Study the drawing (mm; zero at the part's minimum x, y, z) and answer. A direction names the side the tool comes from. Coordinates: 2 decimals unless noted, no trailing zeros. Loops run counter-clockwise (first coordinate to the right, second up) from the corner with the lowest first, then second, coordinate; pieces in that order, holes last. Notation, with made-up numbers: (55, -35.5) -> (64, -35.5) arc R13 ccw to (64, -25.5) -> close; hole circle Ø10 at (58, 55.5). An arc over 180 degrees is marked (long way). Answer as a JSON object with one key per item and string values. Group by question number.
Q1. The part is cut by section A-A on y = 7. Write down the section's boundary in (x, z).
Q2. The part is cut by section D-D on z = 46. Write down the section's boundary in (x, y) (3 decimals), and give its area (3 significant figures).
Q3. Straight lines are drawn through the part: line 1 along Z through (x, y) = (9.25, 2); line 2 along Z through (x, y) = (6.5, 3.75); line 3 along X through (y, z) = (5.5, 14). For each, find the intervals that lie inside material, in ascending order. Write a range as [from, to].
Q4. For the marked faces 1 and 2, determine the directions among +Z, -Z, +X, -X, +Y, -Y from which every point of the face is accessible in a straight line to the end or side of a thin tool.
Q5. The part is cut by section C-C on x = 10.75. Write down the section's boundary in (y, z).
Q6. Each of these flat-tipped pins is pushed along its axis until it touches: P1, Ø3, axis at y = 5.5, z = 29, coming from the -X side (3 decimals); P2, Ø6, axis at x = 3, z = 19, coming from the +Y side (3 decimals); P3, Ø1, axis at x = 2.5, z = 34.5, coming from the +Y side. Where does it stop, or does it pass through?
Q7. The part is cut by section B-B on z = 19. Write down the section's boundary in (x, y) (3 decimals), and give its area (3 significant figures).
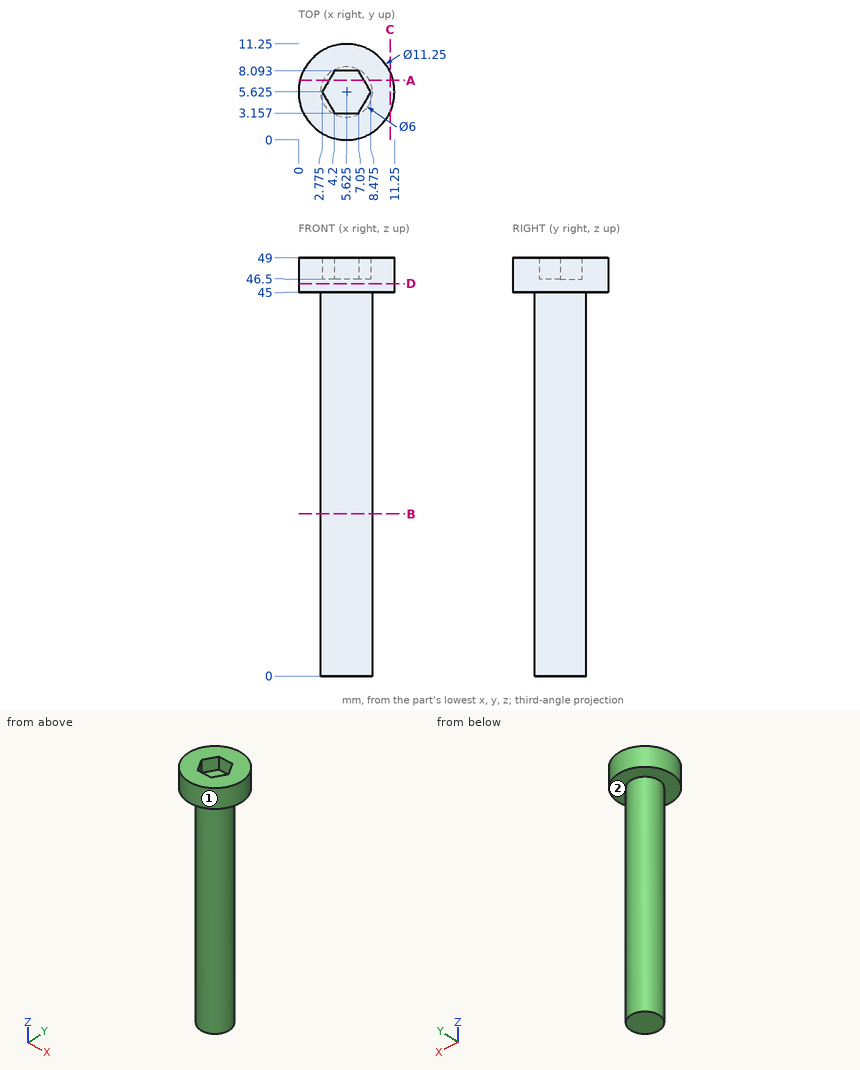
Final values:
{
 "1": {"outline": "(0.17, 45) -> (2.96, 45) -> (2.96, 0) -> (8.29, 0) -> (8.29, 45) -> (11.08, 45) -> (11.08, 49) -> (7.68, 49) -> (7.68, 46.5) -> (3.57, 46.5) -> (3.57, 49) -> (0.17, 49) -> close"},
 "2": {"outline": "circle Ø11.25 at (5.625, 5.625)", "area": "99.4 mm2"},
 "3": {"line 1": "z = [45, 49]", "line 2": "z = [0, 46.5]", "line 3": "x = [2.63, 8.62]"},
 "4": {"face 1": "+Z, -Z", "face 2": "-Z"},
 "5": {"outline": "(3.31, 45) -> (7.94, 45) -> (7.94, 49) -> (3.31, 49) -> close"},
 "6": {"P1": "stops at x = 2.625", "P2": "stops at y = 8.625", "P3": "stops at y = 7.08"},
 "7": {"outline": "circle Ø6 at (5.625, 5.625)", "area": "28.3 mm2"}
}
